```python
from build123d import *

# Parameters (mm, degrees)
F1_DEPTH = 2
F2_DEPTH = 3
F3_DEPTH = 1


with BuildPart() as f1:
    # F0 (on Top) → F1 (new body)
    with BuildSketch(Plane.XY):
        with BuildLine():
            ThreePointArc((-59.7277300679, 28.8946466617), (-59.8627935828, 28.2626599001), (-60.0517619849, 27.6446466617))
            Line((-60.0517619849, 27.6446466617), (-10.0517619849, 27.6446466617))
            Line((-10.0517619849, 27.6446466617), (-10.0517619849, 28.8946466617))
            Line((-10.0517619849, 28.8946466617), (-59.7277300679, 28.8946466617))
        make_face()
        with BuildLine():
            ThreePointArc((-74.5179295257, 28.8946466617), (-67.7684877332, 22.6724899563), (-60.0517619849, 27.6446466617))
            ThreePointArc((-60.0517619849, 27.6446466617), (-59.8627935828, 28.2626599001), (-59.7277300679, 28.8946466617))
            Line((-59.7277300679, 28.8946466617), (-74.5179295257, 28.8946466617))
        make_face()
        with BuildLine():
            ThreePointArc((-74.6228297968, 30.1446466617), (-74.5965587177, 29.5174497096), (-74.5179295257, 28.8946466617))
            Line((-74.5179295257, 28.8946466617), (-59.7277300679, 28.8946466617))
            ThreePointArc((-59.7277300679, 28.8946466617), (-59.6491008759, 29.5174497096), (-59.6228297968, 30.1446466617))
            Line((-59.6228297968, 30.1446466617), (-74.6228297968, 30.1446466617))
        make_face()
    extrude(amount=F1_DEPTH)

    # F0 (on Top) → F2 (join)
    with BuildSketch(Plane.XY):
        with BuildLine():
            ThreePointArc((-74.6228297968, 30.1446466617), (-74.5965587177, 29.5174497096), (-74.5179295257, 28.8946466617))
            Line((-74.5179295257, 28.8946466617), (-59.7277300679, 28.8946466617))
            ThreePointArc((-59.7277300679, 28.8946466617), (-59.6491008759, 29.5174497096), (-59.6228297968, 30.1446466617))
            Line((-59.6228297968, 30.1446466617), (-74.6228297968, 30.1446466617))
        make_face()
        with BuildLine():
            ThreePointArc((-59.6228297968, 30.1446466617), (-59.6491008759, 29.5174497096), (-59.7277300679, 28.8946466617))
            Line((-59.7277300679, 28.8946466617), (-10.0517619849, 28.8946466617))
            Line((-10.0517619849, 28.8946466617), (-10.0517619849, 30.1446466617))
            Line((-10.0517619849, 30.1446466617), (-59.6228297968, 30.1446466617))
        make_face()
    extrude(amount=F2_DEPTH)



with BuildPart() as f1b:
    # F0 (on Top) → F1, piece 2 (new body)
    with BuildSketch(Plane.XY):
        with BuildLine():
            ThreePointArc((-60.0517619849, 32.6446466617), (-67.7684877332, 37.616803367), (-74.5179295257, 31.3946466617))
            Line((-74.5179295257, 31.3946466617), (-59.7277300679, 31.3946466617))
            ThreePointArc((-59.7277300679, 31.3946466617), (-59.8627935828, 32.0266334232), (-60.0517619849, 32.6446466617))
        make_face()
        with BuildLine():
            ThreePointArc((-60.0517619849, 32.6446466617), (-59.8627935828, 32.0266334232), (-59.7277300679, 31.3946466617))
            Line((-59.7277300679, 31.3946466617), (-10.0517619849, 31.3946466617))
            Line((-10.0517619849, 31.3946466617), (-10.0517619849, 32.6446466617))
            Line((-10.0517619849, 32.6446466617), (-60.0517619849, 32.6446466617))
        make_face()
    extrude(amount=F1_DEPTH)


with BuildPart() as f1_1:
    add(f1.part)

    add(f1b.part)  # F3 merges F1b
    # F0 (on Top) → F3 (join)
    with BuildSketch(Plane.XY):
        with BuildLine():
            ThreePointArc((-74.6228297968, 30.1446466617), (-74.5965587177, 29.5174497096), (-74.5179295257, 28.8946466617))
            Line((-74.5179295257, 28.8946466617), (-59.7277300679, 28.8946466617))
            ThreePointArc((-59.7277300679, 28.8946466617), (-59.6491008759, 29.5174497096), (-59.6228297968, 30.1446466617))
            Line((-59.6228297968, 30.1446466617), (-74.6228297968, 30.1446466617))
        make_face()
        with BuildLine():
            ThreePointArc((-74.5179295257, 31.3946466617), (-74.5965587177, 30.7718436138), (-74.6228297968, 30.1446466617))
            Line((-74.6228297968, 30.1446466617), (-59.6228297968, 30.1446466617))
            ThreePointArc((-59.6228297968, 30.1446466617), (-59.6491008759, 30.7718436138), (-59.7277300679, 31.3946466617))
            Line((-59.7277300679, 31.3946466617), (-74.5179295257, 31.3946466617))
        make_face()
        with BuildLine():
            ThreePointArc((-59.7277300679, 31.3946466617), (-59.6491008759, 30.7718436138), (-59.6228297968, 30.1446466617))
            Line((-59.6228297968, 30.1446466617), (-10.0517619849, 30.1446466617))
            Line((-10.0517619849, 30.1446466617), (-10.0517619849, 31.3946466617))
            Line((-10.0517619849, 31.3946466617), (-59.7277300679, 31.3946466617))
        make_face()
    extrude(amount=F3_DEPTH)


solid = f1_1.part
```
Source: CAD feature listing. Evaluate the final solid. Frame: model axes, mm. A direction names the side the tool comes from. Coordinates: 2 decimals unless noted, no trailing zeros. Loops run counter-clockwise (first coordinate to the right, second up) from the corner with the lowest first, then second, coordinate; pieces in that order, holes last. Notation, with made-up numbers: (26, 5) -> (72, 5) arc R9 ccw to (72, 17) -> close; hole circle Ø10 at (82.25, 61). An arc over 180 degrees is marked (long way). One line per item, written item: value. Start each with the question number.
Q1. Set-up query: faces 1 (the face through (-42, 30.145, 2)), 2 (the face through (-42.7, 28.895, 2.5)), 3 (the face through (-52, 32, 2)). Return all of +Z, -Z, +X, -X, +Y, -Y with unobstructed straight access to the full face (end or side cutting, diameter ignored); none if empty.
Q2. Section query B-B, the plane x = -70.5. Return the cut outline in (y, z), and give its area (3 significant figures).
Q3. Line query: line 1 along Y through (x, z) = (-13, 1.1); line 2 along Y through (x, z) = (-47, 2.7); line 3 along Z through (x, y) = (-67.5, 30.5). Output: solid intervals per line, ascending.
Q4. Section query C-C, the plane y = 33.75. Return the cut outline in (x, z), and give its area (3 significant figures).
Q5. Section query A-A, the plane x = -28. Return the cut outline in (y, z), and give its area (3 significant figures).
Q6. Mould query, pull axis Y, two halves, no side actions, for faces 4 (the face through (-35, 32.645, 1)), 5 (the face through (-43, 31, 1)), 6 (the face through (-50, 30, 0)), 7 (the face through (-35, 27.645, 1)). Classes: pulls with the +Y half, pulls with the -Y half, needs draft (parallel to the pull), parting line crosses it, or undercut.
Q7. Contact query for flat-ended pins moving along their axis: P1, Ø0.6, axis at x = -30, z = 2.5, coming from the +Y side; P2, Ø1.5, axis at y = 24.5, z = 2.5, coming from the +X side; P3, Ø7, axis at x = -53, y = 34, coming from the +Z side. Output: stop coordinate, or through.
Q8. Section query D-D, the plane y = 30.75. Return the cut outline in (x, z).
Results:
1. face 1: +Z, +X, -X
1. face 2: +Z, +X, -X, -Y
1. face 3: +Z, +X, -X, +Y
2. outline: (23.45, 0) -> (36.84, 0) -> (36.84, 2) -> (31.39, 2) -> (31.39, 1) -> (30.14, 1) -> (30.14, 3) -> (28.89, 3) -> (28.89, 2) -> (23.45, 2) -> close
2. area: 26.8 mm^2
3. line 1: 27.64 to 30.14, 31.39 to 32.64
3. line 2: 28.89 to 30.14
3. line 3: 0 to 1
4. outline: (-73.7, 0) -> (-60.55, 0) -> (-60.55, 2) -> (-73.7, 2) -> close
4. area: 26.3 mm^2
5. outline: (27.64, 0) -> (32.64, 0) -> (32.64, 2) -> (31.39, 2) -> (31.39, 1) -> (30.14, 1) -> (30.14, 3) -> (28.89, 3) -> (28.89, 2) -> (27.64, 2) -> close
5. area: 10.0 mm^2
6. face 4: pulls with the +Y half
6. face 5: undercut
6. face 6: needs draft
6. face 7: pulls with the -Y half
7. P1: y = 30.14
7. P2: x = -61.61
7. P3: z = 2
8. outline: (-74.6, 0) -> (-10.05, 0) -> (-10.05, 1) -> (-74.6, 1) -> close
